Build history of the part. All positions in model axes, mm. Face numbers are marked on the shaded views. A direction names the side the tool comes from. Round coordinates to 2 decimals unless told otherwise and drop trailing zeros. Write each loop counter-clockwise with the first axis right and the second up, starting at its lowest first coordinate (ties: lowest second). Pieces come first, ordered by that corner, then holes. Notation, with made-up numbers: (0, 2.25) - (11, 2.25) arc R17 ccw to (11, 22.25) - close; hole circle Ø5 at (70.25, 43.25). An arc over 180 degrees is marked (long way). Write each question's results on one line, items separated by ' | '.
from build123d import *

# Parameters (mm, degrees)
ESQUISSE2_R             = 12.439656977
ENL_V_MAT_EXTRU_1_DEPTH = 33.26453161


with BuildPart() as part:
    # Esquisse1 → R_volution1 (revolve)
    with BuildSketch(Plane.XY, mode=Mode.PRIVATE) as r_volution1_sk:
        Polygon((0, 3), (0, 10), (-4, 10), (-4, 0), (25, 0), (25, 2.5), (24.5, 3), align=None)
    revolve(r_volution1_sk.sketch.rotate(Axis((-17.165934066, 0, 0), (1, 0, 0)), 90), axis=Axis((-17.165934066, 0, 0), (1, 0, 0)))

    # Esquisse2 → Enl_v. mat.-Extru.1 (cut, through all)
    with BuildSketch(Plane.ZY.offset(4)):
        Circle(ESQUISSE2_R)
        with BuildLine():
            Line((6.222539674, 7.422539674), (-6.222539674, 7.422539674))
            ThreePointArc((-6.222539674, 7.422539674), (-7.071067812, 7.071067812), (-7.422539674, 6.222539674))
            Line((-7.422539674, 6.222539674), (-7.422539674, -6.222539674))
            ThreePointArc((-7.422539674, -6.222539674), (-7.071067812, -7.071067812), (-6.222539674, -7.422539674))
            Line((-6.222539674, -7.422539674), (6.222539674, -7.422539674))
            ThreePointArc((6.222539674, -7.422539674), (7.071067812, -7.071067812), (7.422539674, -6.222539674))
            Line((7.422539674, -6.222539674), (7.422539674, 6.222539674))
            ThreePointArc((7.422539674, 6.222539674), (7.071067812, 7.071067812), (6.222539674, 7.422539674))
        make_face(mode=Mode.SUBTRACT)
    extrude(amount=-ENL_V_MAT_EXTRU_1_DEPTH, mode=Mode.SUBTRACT)

    # Esquisse3 → Enl_vement de mati_re-R_volution1 (revolve, cut)
    with BuildSketch(Plane.XY, mode=Mode.PRIVATE) as enl_vement_de_mati_re_r_volution1_sk:
        with BuildLine():
            Line((-2.5, 10), (-4.5, 10))
            Line((-4.5, 10), (-4.5, 5.049826293))
            ThreePointArc((-4.5, 5.049826293), (-3.684552713, 7.599477283), (-2.5, 10))
        make_face()
    revolve(enl_vement_de_mati_re_r_volution1_sk.sketch.rotate(Axis((-8.516023748, 0, 0), (1, 0, 0)), 50.025878511), axis=Axis((-8.516023748, 0, 0), (1, 0, 0)), mode=Mode.SUBTRACT)


solid = part.part
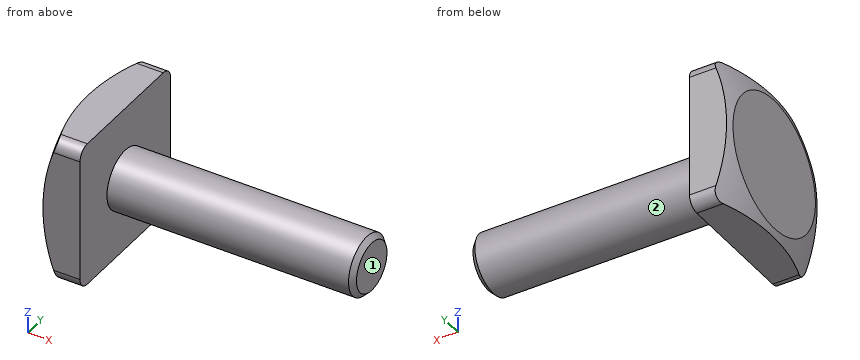
(1) Slice it at A-A, the plane x = 20.5. Write the cut outline in (y, z), and give its area (3 significant figures).
Worked answers:
outline: circle Ø6 at (0, 0) | area: 28.3 mm2
(2) Flat gauge pins, fed straight in: pin 1 Ø4 at (x, y) = (12, -0.5) entering from -Z; pin 2 Ø6 at (x, z) = (20.5, -0.5) entering from -Y; pin 3 Ø1.5 at (y, z) = (-5, 2) entering from +X. Where does each tip first touch, or does it go through?
Worked answers:
pin 1: stops at z = -3 | pin 2: stops at y = -3 | pin 3: stops at x = 0
(3) Tool access for the marked faces 1 and 2: list every direction of +Z, -Z, +X, -X, +Y, -Y with a clear straight run to the whole face (end or side of a thin tool).
Worked answers:
face 1: +Z, -Z, +X, +Y, -Y | face 2: +X
(4) Drill centre lines: probe 1 along X at (y, z) = (2, 6); probe 2 along X at (y, z) = (4, -6.25); probe 3 along Y at (x, z) = (21, -1.5). Where is each one in solid material? Low to high. Write a range as [from, to].
Worked answers:
probe 1: x = [-4, 0] | probe 2: x = [-3.76, 0] | probe 3: y = [-2.6, 2.6]
